Part print with two shaded views. Sizes in mm from the minimum x, y, z corner. Give positions to 0.01 mm unless a question says otherwise; leave off trailing zeros. Write each loop counter-clockwise with the first axis right and the second up, starting at its lowest first coordinate (ties: lowest second). Pieces come first, ordered by that corner, then holes. Notation, with made-up numbers: (-1.5, -26) - (36.5, -26) arc R26 ccw to (36.5, 7) - close; hole circle Ø5 at (65.5, 46.5). An arc over 180 degrees is marked (long way). One line per item, written item: value. Start each with the question number.
(1) Probe L1, parallel to Y at x = 9.5, z = 17.4; L2, parallel to Y at x = 134.5, z = 11.5; L3, parallel to Y at x = 72, z = 11. List the from-to ranges inside material, lowest first.
(2) Cut at A-A, the plane y = 53. List the corners of the cut face in (x, z), and give its area (3 significant figures).
(3) Drop a flat-ended pin along its axis: P1, Ø4.5, axis at x = 46.5, y = 8.83, coming from the +Z side. Give the stop position or say it passes through.
(4) Cut at C-C, the plane y = 18. List the corners of the cut face in (x, z).
(5) Mould opens along X. For the marked faces 1, 2 and 3 say: pulls with the +X half, pulls with the -X half, needs draft (parallel to the pull), parting line crosses it, or undercut.
(6) Cut at D-D, the plane x = 123. List the corners of the cut face in (y, z).
(7) Cut at B-B, the plane x = 46.5. List the corners of the cut face in (y, z).
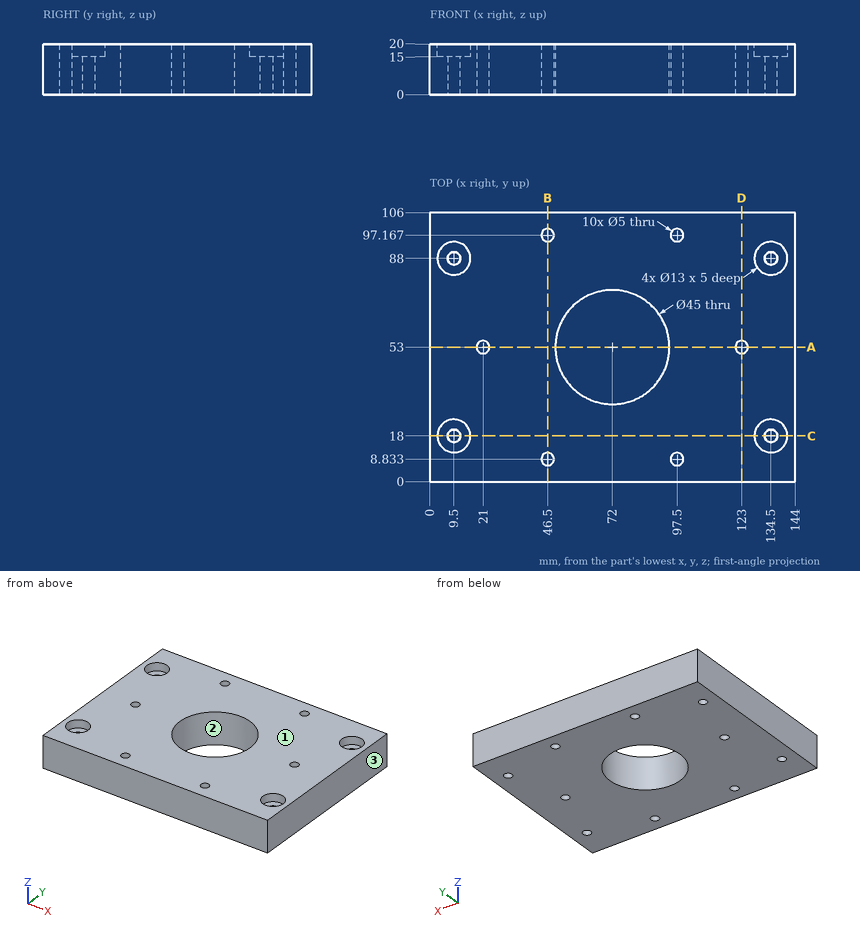
Answers follow:
1. L1: y = 0 to 11.5, 24.5 to 81.5, 94.5 to 106
1. L2: y = 0 to 15.5, 20.5 to 85.5, 90.5 to 106
1. L3: y = 0 to 30.5, 75.5 to 106
2. outline: (0, 0) - (18.5, 0) - (18.5, 20) - (0, 20) - close; (23.5, 0) - (49.5, 0) - (49.5, 20) - (23.5, 20) - close; (94.5, 0) - (120.5, 0) - (120.5, 20) - (94.5, 20) - close; (125.5, 0) - (144, 0) - (144, 20) - (125.5, 20) - close
2. area: 1,780 mm²
3. P1: passes through
4. outline: (0, 0) - (7, 0) - (7, 15) - (3, 15) - (3, 20) - (0, 20) - close; (12, 0) - (132, 0) - (132, 15) - (128, 15) - (128, 20) - (16, 20) - (16, 15) - (12, 15) - close; (137, 0) - (144, 0) - (144, 20) - (141, 20) - (141, 15) - (137, 15) - close
5. face 1: needs draft
5. face 2: undercut
5. face 3: pulls with the +X half
6. outline: (0, 0) - (50.5, 0) - (50.5, 20) - (0, 20) - close; (55.5, 0) - (106, 0) - (106, 20) - (55.5, 20) - close
7. outline: (0, 0) - (6.33, 0) - (6.33, 20) - (0, 20) - close; (11.33, 0) - (94.67, 0) - (94.67, 20) - (11.33, 20) - close; (99.67, 0) - (106, 0) - (106, 20) - (99.67, 20) - close
